Could you check a few things on this model? Use its own coordinates, in mm. A direction names the side the tool comes from. Coordinates: 2 decimals unless noted, no trailing zeros. Loops run counter-clockwise (first coordinate to the right, second up) from the corner with the lowest first, then second, coordinate; pieces in that order, holes last.
1) For faces 1 (the face through (216, 340, 0)), 2 (the face through (-10.586, 815.477, 22.148)), 3 (the face through (-205.856, -124.989, 22.148)), 4 (the face through (184.05, 353.67, 22.15)), 5 (the face through (199.46, 331.83, 4.51)), which set-ups out of +Z, -Z, +X, -X, +Y, -Y let a thin tool reach every point of the face, with its end or its side?
2) If I drill on line 1 along Z through (x, y) = (226.5, 319); line 2 along Y through (x, z) = (-95, 19); line 3 along Y through (x, z) = (341, 10.5), over which ranges is the centre line in solid material (lowest first)?
3) Imagine slicing it at A-A on x = -96.5. Please give me the cut outline in (y, z).
4) Will these pins go through, and if not, where does the flat tip stop? P1, Ø12.5, axis at x = -220.65, y = -125.43, coming from the -Z side; P2, Ø10, axis at x = -213, y = -127.5, coming from the +Z side; P3, Ø6, axis at x = 103.5, z = 11, coming from the +Y side; P4, Ø4.5, axis at x = 74.5, z = 24.5, coming from the +Y side.
5) Thinking about a two-plate mould opening in Z: for faces 6 (the face through (-220, -133, 15)), 7 (the face through (243.191, 333.922, 22.148)), 8 (the face through (-233.833, -123.164, 7.524)), which applies, released by +Z, released by -Z, zero draft, split by the parting line, or undercut?
6) Imagine slicing it at B-B on z = 63. Please give me the cut outline in (x, y).
```python
from build123d import *

# Parameters (mm, degrees)
BOSS_EXTRUDE1_DEPTH = 44.5
FILLET2_R           = 15
SKETCH2_R           = 7
CUT_EXTRUDE1_DEPTH  = 14
SKETCH3_R           = 7
CUT_EXTRUDE2_DEPTH  = 14
SKETCH4_R           = 7
CUT_EXTRUDE3_DEPTH  = 14
SKETCH5_R           = 7
CUT_EXTRUDE4_DEPTH  = 952.271625519
SKETCH6_W           = 14.5
SKETCH6_H           = 44.5
CUT_EXTRUDE5_DEPTH  = 936.632574619
BOSS_EXTRUDE3_DEPTH = 40


with BuildPart() as part:
    # Sketch1 → Boss-Extrude1 (new body)
    with BuildSketch(Plane.XY):
        Polygon((-253.518736915, -141.579738071), (475.109189289, -141.579738071), (4.687860899, 822.926918688), (-35.308474161, 803.419402656), (409.63823983, -108.856554338), (-223.36176017, -108.856554338), align=None)
    extrude(amount=BOSS_EXTRUDE1_DEPTH)

    # Fillet2
    fillet2_edges = [part.edges().sort_by_distance(p)[0] for p in [
        (239.898525094, 340.673590309, 44.5),
        (-15.310306631, 813.173160672, 44.5),
        (187.164882834, 347.281424159, 44.5),
        (93.13823983, -108.856554338, 44.5),
        (-238.440248543, -125.218146204, 44.5),
        (93.13823983, -108.856554338, 0),
        (187.164882834, 347.281424159, 0),
        (-15.310306631, 813.173160672, 0),
        (239.898525094, 340.673590309, 0),
        (110.795226187, -141.579738071, 0),
        (-238.440248543, -125.218146204, 0),
        (110.795226187, -141.579738071, 44.5),
    ]]
    fillet(fillet2_edges, radius=FILLET2_R)

    # Sketch2 → Cut-Extrude1 (cut)
    with BuildSketch(Plane(origin=(-323.336767908, 662.938617367, 0), x_dir=(0.8987940462991654, 0.43837114678908073, 0), z_dir=(-0.43837114678908073, 0.8987940462991654, 0))):
        with Locations(Location((339.470196695, -21.913602874, 0), (0, 0, 180))):
            Circle(SKETCH2_R)
    extrude(amount=-CUT_EXTRUDE1_DEPTH, mode=Mode.SUBTRACT)

    # Sketch3 → Cut-Extrude2 (cut)
    with BuildSketch(Plane(origin=(-66.534083276, 61.316368798, 0), x_dir=(0, 0, 1), z_dir=(-0.735352443447444, 0.6776848706558778, 0))):
        with Locations(Location((22.366337019, -255.510068241, 0), (0, 0, 270))):
            Circle(SKETCH3_R)
    extrude(amount=-CUT_EXTRUDE2_DEPTH, mode=Mode.SUBTRACT)

    # Sketch4 → Cut-Extrude3 (cut)
    with BuildSketch(Plane(origin=(0, -141.579738071, 0), x_dir=(-1, 0, 0), z_dir=(0, -1, 0))):
        with Locations(Location((233.419507196, -21.201481555, 0), (0, 0, 117.634316404))):
            Circle(SKETCH4_R)
    extrude(amount=-CUT_EXTRUDE3_DEPTH, mode=Mode.SUBTRACT)

    # Sketch5 → Cut-Extrude4 (cut, through all)
    with BuildSketch(Plane.XY.offset(44.5)):
        with Locations(Location((-220.649115428, -125.427110978, 0), (0, 0, 350.522457382))):
            Circle(SKETCH5_R)
    extrude(amount=-CUT_EXTRUDE4_DEPTH, mode=Mode.SUBTRACT)

    # Sketch6 → Cut-Extrude5 (cut, through all)
    with BuildSketch(Plane(origin=(-66.534083276, 61.316368798, 0), x_dir=(0, 0, 1), z_dir=(-0.735352443447444, 0.6776848706558778, 0))):
        with Locations((22.25, -253.666818768)):
            Rectangle(SKETCH6_W, SKETCH6_H)
    extrude(amount=-CUT_EXTRUDE5_DEPTH, mode=Mode.SUBTRACT)

    # Sketch8 → Boss-Extrude3 (add)
    with BuildSketch(Plane.XY.offset(44.5)):
        with BuildLine():
            ThreePointArc((350.492241226, 46.628294304), (357.703100488, 46.229913436), (361.428471817, 52.416738718))
            ThreePointArc((361.428471817, 52.416738718), (354.659562876, 59.412923172), (347.443729839, 52.878668912))
            Line((347.443729839, 52.878668912), (350.492241226, 46.628294304))
        make_face()
        with BuildLine():
            Line((350.492241226, 46.628294304), (347.443729839, 52.878668912))
            ThreePointArc((347.443729839, 52.878668912), (348.136913493, 49.34814069), (350.492241226, 46.628294304))
        make_face()
    extrude(amount=BOSS_EXTRUDE3_DEPTH)


solid = part.part
```
Filled in:
1. face 1: -Z, +X, -X, +Y, -Y
1. face 2: +Z, -Z, -X, +Y
1. face 3: -X, -Y
1. face 4: +Z, -Z, -X
1. face 5: -Z, -X
2. line 1: z = 0 to 44.5
2. line 2: y = -141.58 to -108.86
2. line 3: y = -140.89 to -109.55, 33.45 to 131.81
3. outline: (-141.58, 15) arc R15 ccw to (-126.58, 0) - (-123.86, 0) arc R15 ccw to (-108.86, 15) - (-108.86, 29.5) arc R15 ccw to (-123.86, 44.5) - (-126.58, 44.5) arc R15 ccw to (-141.58, 29.5) - close
4. P1: passes through
4. P2: stops at z = 44.5
4. P3: stops at y = 625.48
4. P4: stops at y = 684.4
5. face 6: undercut
5. face 7: zero draft
5. face 8: released by -Z
6. outline: circle Ø14 at (354.43, 52.42)
